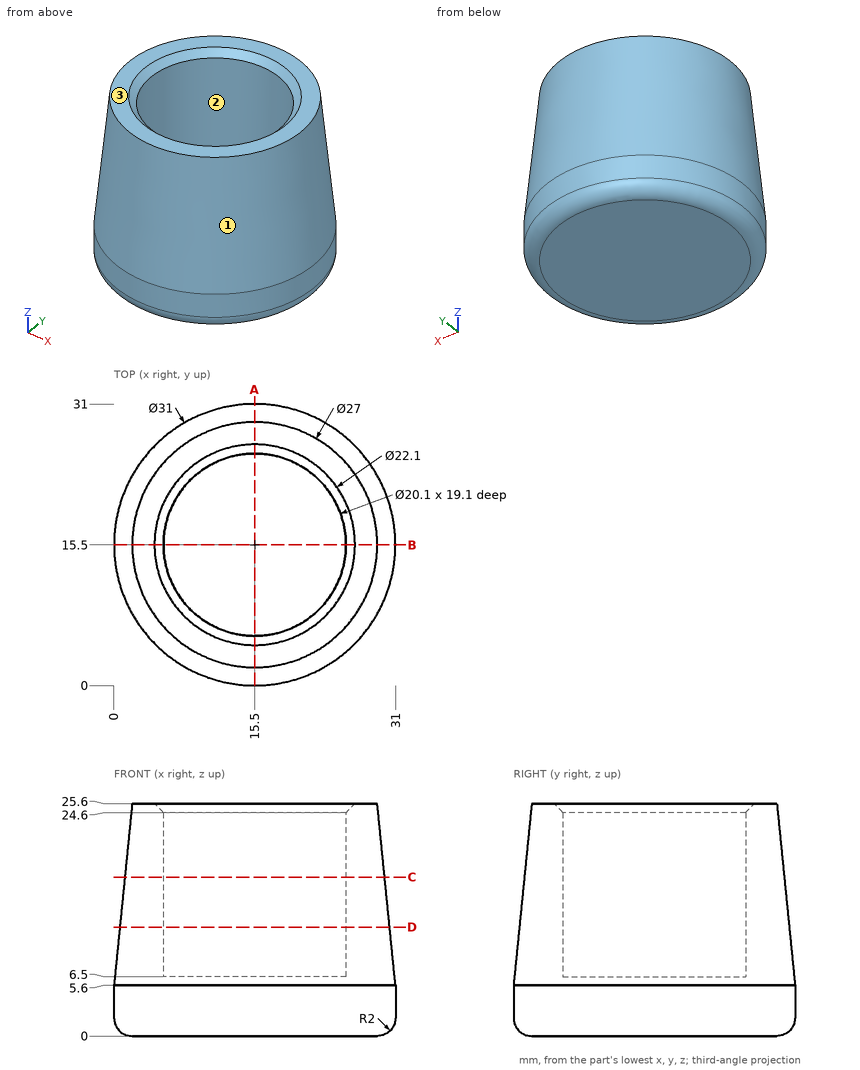
Part print with two shaded views. Sizes in mm from the minimum x, y, z corner. Round coordinates to 2 decimals unless told otherwise and drop trailing zeros. Order: outer loops, then holes, each group sorted by start corner. A loop starts at its lowest first (then second) coordinate and runs counter-clockwise, first axis right, second up. Notation, with made-up numbers: M 28,32.5 L 84,32.5 A17 ccw 84,55.5 Z; hole C 54,17 d2. An arc over 180 degrees is marked long. Put each result on its own line as item: value. Start each with the question number.
1. Slice it at D-D on z = 12. List the corners of the cut face in (x, y).
2. Two-plate mould, pull along Y, no slides. Class the marked faces 1, 2 and 3: +Y half, -Y half, draft (parallel to the pull), parting line (faces both ways), or undercut.
3. Slice it at A-A on x = 15.5. List the corners of the cut face in (y, z).
4. Drill centre lines: probe 1 along Z at (x, y) = (12, 11); probe 2 along Y at (x, z) = (14, 22.25); probe 3 along X at (y, z) = (15.5, 12). Where is each one in solid material? Low to high. Write a range as [from, to].
5. Drop flat-ended pins along their axis: pin 1 (4 mm diameter, centred on x = 11.5, z = 11.5, fed in from +Y); pin 2 (12 mm diameter, centred on y = 6, z = 15, fed in from -X); pin 3 (5 mm diameter, centred on x = 19.5, z = 22, fed in from -Y). Give the stop position or say it passes through.
6. Slice it at C-C on z = 17.5. List the corners of the cut face in (x, y), then the cut area to 3 significant figures.
Findings:
1. outline: C 15.5,15.5 d29.72; hole C 15.5,15.5 d20.1
2. face 1: parting line
2. face 2: undercut
2. face 3: draft
3. outline: M 0,2 A2 ccw 2,0 L 29,0 A2 ccw 31,2 L 31,5.6 L 29,25.6 L 26.55,25.6 L 25.55,24.6 L 25.55,6.5 L 5.45,6.5 L 5.45,24.6 L 4.45,25.6 L 2,25.6 L 0,5.6 Z
4. probe 1: [0, 6.5]
4. probe 2: [1.75, 5.56], [25.44, 29.25]
4. probe 3: [0.64, 5.45], [25.55, 30.36]
5. pin 1: y = 30.34
5. pin 2: x = 1.25
5. pin 3: y = 1.63
6. outline: C 15.5,15.5 d28.62; hole C 15.5,15.5 d20.1
6. area: 326 mm2
